Input: part model. Units: mm. Frame: model coordinates. Face numbers are marked on the shaded views. Give positions to 0.01 mm unless a question says otherwise; leave off trailing zeros. Loops run counter-clockwise (first coordinate to the right, second up) from the corner with the lowest first, then second, coordinate; pieces in that order, holes last.
from build123d import *

# Parameters (mm, degrees)
EXTRUDE_THIN1_DEPTH = 17.5005


with BuildPart() as part:
    # Sketch1 → Extrude-Thin1 (new body, symmetric)
    with BuildSketch(Plane.XY):
        Polygon((0, 0), (200, 0), (200, 40), (220, 40), (220, -20), (0, -20), align=None)
    extrude_thin1 = extrude(amount=EXTRUDE_THIN1_DEPTH, both=True)

    # Mirror1: Extrude-Thin1 across plane
    add(extrude_thin1.mirror(Plane(origin=(0, 0, 0), x_dir=(0, 0, 1), z_dir=(1, 0, 0))))


solid = part.part
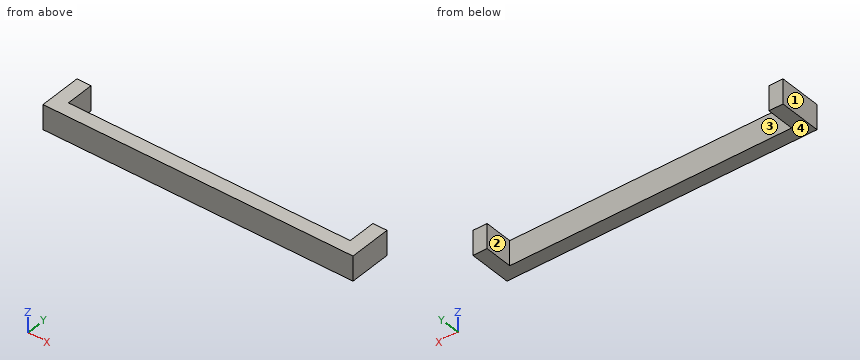
(1) Ray query, probe 1 along X at (y, z) = (6.5, -2); probe 2 along Y at (x, z) = (-109, -5). Return the intervals inside material, ascending.
Values follow:
probe 1: x = -220 to -200, 200 to 220
probe 2: y = -20 to 0
(2) Cut plane B-B (z = 13.5). Return the cut outline in (x, y).
Values follow:
outline: (-220, -20) - (220, -20) - (220, 40) - (200, 40) - (200, 0) - (-200, 0) - (-200, 40) - (-220, 40) - close
(3) Pin query (flat end, axial travel): pin 1 Ø17.5 at (x, z) = (85.5, -8.5) entering from +Y; pin 2 Ø6 at (x, y) = (104, 1.5) entering from +Z. Return the tip coordinate at first contact, or that it passes through.
Values follow:
pin 1: stops at y = 0
pin 2: stops at z = 17.5
(4) Cut plane A-A (y = 34.5). Return the cut outline in (x, z).
Values follow:
outline: (-220, -17.5) - (-200, -17.5) - (-200, 17.5) - (-220, 17.5) - close; (200, -17.5) - (220, -17.5) - (220, 17.5) - (200, 17.5) - close
(5) Cut plane C-C (x = -182). Return the cut outline in (y, z), and give its area (3 significant figures).
Values follow:
outline: (-20, -17.5) - (0, -17.5) - (0, 17.5) - (-20, 17.5) - close
area: 700 mm2
(6) Mould query, pull axis X, two halves, no side actions, for the marked faces 1, 2, 3 and 4. Classes: +X half, -X half, draft (parallel to the pull), parting line (faces both ways), or undercut.
Values follow:
face 1: -X half
face 2: undercut
face 3: undercut
face 4: draft
